Can you work these out from the model? Positions are in its coordinate system, mm. Face numbers are marked on the shaded views. A direction names the side the tool comes from. Coordinates: 2 decimals unless noted, no trailing zeros. Order: outer loops, then holes, each group sorted by start corner. A loop starts at its lowest first (then second) coordinate and runs counter-clockwise, first axis right, second up. Notation, with made-up numbers: (83, -36) -> (137, -36) arc R21 cw to (137, -23) -> close; hole circle Ø10 at (3, 10). An arc over 180 degrees is marked (long way). Write item = value, one per line.
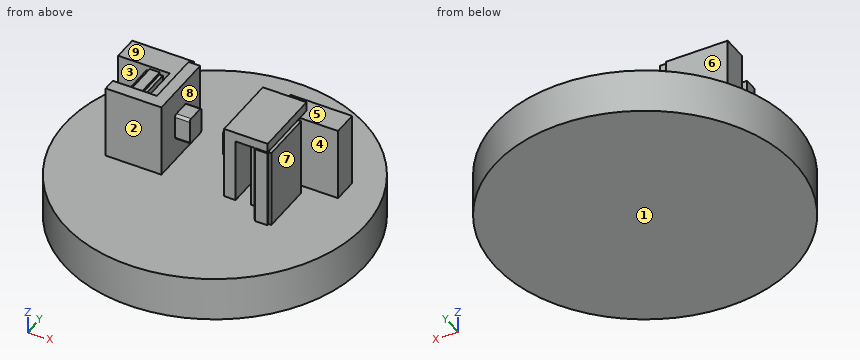
```python
from build123d import *

# Parameters (mm, degrees)
SKETCH_1_R             = 30.549115646
EXTRUDE_1_DEPTH        = 9
EXTRUDE_2_DEPTH        = 15
SKETCH_8_W             = 2.353970865
SKETCH_8_H             = 15
EXTRUDE_3_DEPTH        = 8
EXTRUDE_3_2_DEPTH      = 8
SKETCH_12_W            = 2.353970865
SKETCH_12_H            = 15
EXTRUDE_5_DEPTH        = 6
EXTRUDE_START          = -8.741924
SKETCH_14_W            = 15
SKETCH_14_H            = 2.566345669
EXTRUDE_7_DEPTH        = 9
SKETCH_15_W            = 6.541100851
SKETCH_15_H            = 1.915380037
EXTRUDE_8_DEPTH        = 6
SKETCH_15_2_W          = 6.541100851
SKETCH_15_2_H          = 1.915380037
EXTRUDE_9_DEPTH        = 8
EXTRUDE_10_DEPTH       = 16.020510359
EXTRUDE_11_DEPTH       = 12.778725016
SKETCH_19_W            = 5.407207082
SKETCH_19_H            = 4.197700235
EXTRUDE_12_DEPTH       = 3
FILLET_1_R             = 0.5
FILLET_1_OF_MIRROR_4_R = 0.5


with BuildPart() as part:
    # Sketch 1 → Extrude 1 (new body)
    with BuildSketch(Plane.XY):
        Circle(SKETCH_1_R)
    extrude(amount=EXTRUDE_1_DEPTH)

    # Sketch 3 → Extrude 2 (add)
    with BuildSketch(Plane.XY.offset(9)):
        Polygon((-22.413460509, 4.778725016), (-11.904585252, 4.778725016), (-11.904585252, -4.489323984), (-9.852070554, -4.489323984), (-9.852070554, 7.306952327), (-9.852070554, 9.852070554), (-22.413460509, 9.852070554), align=None)
        Polygon((22.413460509, 9.852070554), (9.852070554, 9.852070554), (9.852070554, 7.306952327), (9.852070554, -4.489323984), (11.904585252, -4.489323984), (11.904585252, 4.778725016), (22.413460509, 4.778725016), align=None)
    extrude(amount=EXTRUDE_2_DEPTH)



with BuildPart() as body_2:
    # Sketch 8 → Extrude 3 (new body)
    with BuildSketch(Plane(origin=(0, 0, 0), x_dir=(1, 0, 0), z_dir=(0, 1, 0))):
        with Locations((-7.564938163, -19.435890396)):
            Rectangle(SKETCH_8_W, SKETCH_8_H)
    extrude(amount=-EXTRUDE_3_DEPTH)



with BuildPart() as body_3:
    # Sketch 8 → Extrude 3 2 (new body)
    with BuildSketch(Plane(origin=(0, 0, 0), x_dir=(1, 0, 0), z_dir=(0, 1, 0))):
        with Locations((7.564938163, -19.435890396)):
            Rectangle(SKETCH_8_W, SKETCH_8_H)
    extrude(amount=-EXTRUDE_3_2_DEPTH)


with BuildPart() as body_2_1:
    add(body_2.part)

    add(body_3.part)  # Extrude 5 merges body 3
    # Sketch 12 → Extrude 5 (add)
    with BuildSketch(Plane(origin=(0, 0, 0), x_dir=(1, 0, 0), z_dir=(0, 1, 0))):
        with Locations((-7.564938163, -19.435890396)):
            Rectangle(SKETCH_12_W, SKETCH_12_H)
        with Locations((7.564938163, -19.435890396)):
            Rectangle(SKETCH_12_W, SKETCH_12_H)
    extrude(amount=EXTRUDE_5_DEPTH)


with BuildPart() as extrude_7_tool:
    # Sketch 14 → Extrude 7 (new body)
    with BuildSketch(Plane(origin=(0, 0, 0), x_dir=(0, 0, -1), z_dir=(1, 0, 0)).offset(EXTRUDE_START)):
        with Locations((-19.435890396, -6.716827165)):
            Rectangle(SKETCH_14_W, SKETCH_14_H)
    extrude(amount=-EXTRUDE_7_DEPTH)


with BuildPart() as body_2_2:
    add(body_2_1.part)


with BuildPart() as body_2_3:
    # Extrude 7: joined with extrude_7_tool
    add(body_2_2.part.fuse(extrude_7_tool.part, tol=0.00001))

    # Sketch 15 → Extrude 8 (add)
    with BuildSketch(Plane(origin=(0, 0, 0), x_dir=(1, 0, 0), z_dir=(0, 1, 0))):
        with Locations((12.012474021, -25.978200378)):
            Rectangle(SKETCH_15_W, SKETCH_15_H)
    extrude(amount=EXTRUDE_8_DEPTH)

    # Sketch 15_2 → Extrude 9 (add)
    with BuildSketch(Plane(origin=(0, 0, 0), x_dir=(1, 0, 0), z_dir=(0, 1, 0))):
        with Locations((12.012474021, -25.978200378)):
            Rectangle(SKETCH_15_2_W, SKETCH_15_2_H)
    extrude(amount=-EXTRUDE_9_DEPTH)


with BuildPart() as part_1:
    add(part.part)

    add(body_2_3.part)  # Extrude 10 merges body 2
    # Sketch 16 → Extrude 10 (add)
    with BuildSketch(Plane.XY.offset(9)):
        Polygon((15.402096143, -7.866023052), (15.954530634, -7.866023052), (15.954530634, 2.891816022), (15.402096143, 2.891816022), (15.402096143, 3.244620079), (12.852605538, 3.244620079), (12.852605538, 2.891816022), (12.56859722, 2.891816022), (12.56859722, -7.866023052), (12.852605538, -7.866023052), (12.852605538, -8.286124494), (15.402096143, -8.286124494), align=None)
    extrude(amount=EXTRUDE_10_DEPTH)

    # Sketch 18 → Extrude 11 (add)
    with BuildSketch(Plane.XZ.offset(-4.778725016)):
        Polygon((-15.980879444, 13.400073381), (-16.608948942, 13.400073381), (-16.608948942, 22.960686847), (-15.980879444, 22.960686847), (-15.980879444, 23.449185345), (-13.957099951, 23.449185345), (-13.957099951, 22.960686847), (-13.329030453, 22.960686847), (-13.329030453, 13.400073381), (-13.957099951, 13.400073381), (-13.957099951, 13.108195893), (-15.980879444, 13.108195893), align=None)
    extrude(amount=EXTRUDE_11_DEPTH)

    # Sketch 19 → Extrude 12 (add)
    with BuildSketch(Plane(origin=(-6.38795273, 0, 0), x_dir=(0, 0, -1), z_dir=(1, 0, 0))):
        with Locations((-19.241101822, -0.973659034)):
            Rectangle(SKETCH_19_W, SKETCH_19_H)
    extrude_12 = extrude(amount=EXTRUDE_12_DEPTH)

    # Fillet 1
    fillet_1_edges = [part_1.edges().sort_by_distance(p)[0] for p in [
        (-4.88795273, 1.125191084, 21.944705363),
        (-4.88795273, -3.072509151, 21.944705363),
        (-4.88795273, -3.072509151, 16.537498281),
        (-4.88795273, 1.125191084, 16.537498281),
    ]]
    fillet(fillet_1_edges, radius=FILLET_1_R)

    # Mirror 4: Extrude 12 across plane
    add(extrude_12.mirror(Plane(origin=(0, 0, 0), x_dir=(0, 0, 1), z_dir=(1, 0, 0))))

    # Fillet 1 of Mirror 4
    fillet_1_of_mirror_4_edges = [part_1.edges().sort_by_distance(p)[0] for p in [
        (4.88795273, 1.125191084, 21.944705363),
        (4.88795273, -3.072509151, 21.944705363),
        (4.88795273, -3.072509151, 16.537498281),
        (4.88795273, 1.125191084, 16.537498281),
    ]]
    fillet(fillet_1_of_mirror_4_edges, radius=FILLET_1_OF_MIRROR_4_R)


solid = part_1.part
```
Item 1: For the marked faces 5, 6, 7, 8 and 9, which set-ups out of +Z, -Z, +X, -X, +Y, -Y let a thin tool reach every point of the face, with its end or its side?
A:
face_5 = +Y
face_6 = +Z, +X, -X, +Y
face_7 = +Z, +X, -Y
face_8 = none
face_9 = +Z, -X, +Y
Item 2: I want a section at C-C, the plane z = 3.75. Please give me the cut outline in (x, y).
A:
outline = circle Ø61.1 at (0, 0)
Item 3: I want a section at A-A, the plane x = -11. Please give me the cut outline in (y, z).
A:
outline = (-28.5, 0) -> (28.5, 0) -> (28.5, 9) -> (9.85, 9) -> (9.85, 24) -> (-4.49, 24) -> (-4.49, 9) -> (-28.5, 9) -> close; (-8, 11.94) -> (-5.43, 11.94) -> (-5.43, 26.94) -> (-8, 26.94) -> close
Item 4: I want a section at D-D, the plane y = -12. Please give me the cut outline in (x, z), plus the area to 3 significant figures.
A:
outline = (-28.09, 0) -> (28.09, 0) -> (28.09, 9) -> (-28.09, 9) -> close
area = 506 mm2
Item 5: I want a section at B-B, the plane x = -20.5. Please give me the cut outline in (y, z).
A:
outline = (-22.65, 0) -> (22.65, 0) -> (22.65, 9) -> (9.85, 9) -> (9.85, 24) -> (4.78, 24) -> (4.78, 9) -> (-22.65, 9) -> close
Item 6: If we mould it in two halves opening along Y, with no side actions, what happens to the marked faces 1, 2, 3 and 4? For each: pulls with the +Y half, pulls with the -Y half, needs draft (parallel to the pull), parting line crosses it, or undercut.
A:
face_1 = needs draft
face_2 = pulls with the -Y half
face_3 = undercut
face_4 = undercut
Item 7: I'm going to push flat-ended pins straight in: P1, Ø6, axis at x = 19.5, y = 23, coming from the -Z side; P2, Ø10, axis at x = -10, z = 8, coming from the +Y side; P3, Ø12, axis at x = -22, y = -19.5, coming from the +Z side; P4, Ø2.5, axis at x = 11, z = 15.5, coming from the -Y side. Where does each tip first touch, or does it pass through?
A:
P1 = 0
P2 = 30.14
P3 = 9
P4 = -4.49
Item 8: If I drill on probe 1 along X at (y, z) = (-5.5, 18); probe 2 along X at (y, z) = (9.5, 19.25); probe 3 along Y at (x, z) = (15, 10.25), over which ranges is the centre line in solid material (lowest first)?
A:
probe_1 = -17.74 to -6.39, 6.39 to 8.74, 12.57 to 15.95
probe_2 = -22.41 to -9.85, 9.85 to 22.41
probe_3 = -8.29 to 3.24, 4.78 to 9.85
